Geometry: final body of the model. Coordinates: model frame, mm. Face numbers are marked on the shaded views. A direction names the side the tool comes from. Give positions to 0.01 mm unless a question says otherwise; leave off trailing zeros. Write each loop counter-clockwise with the first axis right and the second up, starting at its lowest first coordinate (ties: lowest second). Pieces come first, ordered by that corner, then holes. Notation, with made-up numbers: M -19,-21.75 L 29,-21.75 A22 ccw 29,-11.75 Z; hole C 46,48.5 d5. An arc over 180 degrees is marked long. Answer as a JSON object with one key per item and string values.
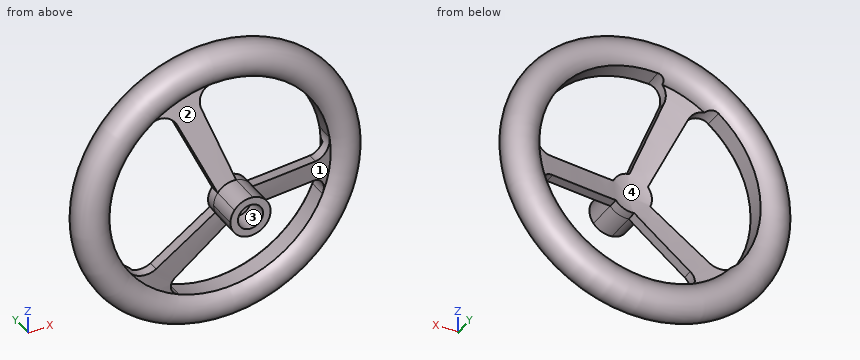
from build123d import *

# Parameters (mm, degrees)
CUT_EXTRUDE1_DEPTH = 218.993055499


with BuildPart() as part:
    # Sketch1 → Revolve1 (revolve)
    with BuildSketch(Plane.XY, mode=Mode.PRIVATE) as revolve1_sk:
        with BuildLine():
            Line((20, -100.740243091), (20, -69.715325618))
            Line((20, -69.715325618), (110.198752068, -44.459675039))
            ThreePointArc((110.198752068, -44.459675039), (141.851870345, -30.404499927), (107.502452813, -34.830034842))
            Line((107.502452813, -34.830034842), (0, -64.930721629))
            Line((0, -64.930721629), (0, -78.058110007))
            Line((0, -78.058110007), (12.5, -78.058110007))
            Line((12.5, -78.058110007), (12.5, -100.740243091))
            Line((12.5, -100.740243091), (20, -100.740243091))
        make_face()
    revolve(revolve1_sk.sketch.rotate(Axis((0, 122.203800038, 0), (0, -1, 0)), 180), axis=Axis((0, 122.203800038, 0), (0, -1, 0)))

    # Sketch3 → Cut-Extrude1 (cut, through all)
    with BuildSketch(Plane.XZ.offset(100.740243091)):
        with BuildLine():
            Line((-15.982116295, 12.023807996), (-45.159681095, 80.612688819))
            ThreePointArc((-45.159681095, 80.612688819), (-55.246837021, 89.273395117), (-68.253125072, 86.51748884))
            ThreePointArc((-68.253125072, 86.51748884), (-109.03897279, 15.945763394), (-90.169598509, -63.349889203))
            ThreePointArc((-90.169598509, -63.349889203), (-78.581603296, -69.711168161), (-66.461068877, -64.43479171))
            Line((-66.461068877, -64.43479171), (-18.403981322, -7.82901472))
            ThreePointArc((-18.403981322, -7.82901472), (-19.852822716, 2.421865027), (-15.982116295, 12.023807996))
        make_face()
        with BuildLine():
            Line((15.982116295, -12.023807996), (89.970611905, -21.04973607))
            ThreePointArc((89.970611905, -21.04973607), (101.087630383, -28.341543009), (102.04423972, -41.602140538))
            ThreePointArc((102.04423972, -41.602140538), (43.137382604, -101.40478874), (-40.799780672, -102.36768462))
            ThreePointArc((-40.799780672, -102.36768462), (-49.689609543, -92.481861898), (-47.232795837, -79.415775465))
            Line((-47.232795837, -79.415775465), (-2.421865027, -19.852822716))
            ThreePointArc((-2.421865027, -19.852822716), (7.82901472, -18.403981322), (15.982116295, -12.023807996))
        make_face()
        with BuildLine():
            Line((2.421865027, 19.852822716), (-21.185241198, 90.169588344))
            ThreePointArc((-21.185241198, 90.169588344), (-19.455713432, 103.249492349), (-8.062704922, 109.903401888))
            ThreePointArc((-8.062704922, 109.903401888), (69.001859108, 85.921524643), (109.052905743, 15.85019578))
            ThreePointArc((109.052905743, 15.85019578), (104.936446564, 3.208466781), (92.392476932, -1.196913354))
            Line((92.392476932, -1.196913354), (18.403981322, 7.82901472))
            ThreePointArc((18.403981322, 7.82901472), (12.023807996, 15.982116295), (2.421865027, 19.852822716))
        make_face()
    extrude(amount=-CUT_EXTRUDE1_DEPTH, mode=Mode.SUBTRACT)


solid = part.part
1) Contact query for flat-ended pins moving along their axis: P1, Ø3, axis at x = -10.5, y = -79.5, coming from the +Z side; P2, Ø5, axis at x = -88, y = -26, coming from the +Z side; P3, Ø3, axis at y = -46.5, z = 89, coming from the +X side. Output: stop coordinate, or through.
Geometry check:
{"P1": "stops at z = 17.86", "P2": "stops at z = 111.42", "P3": "stops at x = 107.83"}
2) Cut plane B-B on z = -60. Give the number of separate pieces and of enclosed holes in the cut face, and give its area (3 significant figures).
Geometry check:
{"separate pieces": "3", "enclosed holes": "0", "area": "2,430 mm2"}
3) Set-up query: the marked faces 3 and 4. Return all of +Z, -Z, +X, -X, +Y, -Y with unobstructed straight access to the full face (end or side cutting, diameter ignored); none if empty.
Geometry check:
{"face 3": "-Y", "face 4": "+Y"}
4) Pull-direction query (X, two-part tool) for the marked faces 1 and 2; classes: pulls with the +X half, pulls with the -X half, needs draft (parallel to the pull), parting line crosses it, or undercut.
Geometry check:
{"face 1": "undercut", "face 2": "undercut"}
5) Line query: line 1 (Z direction, x = 0, y = -86.25); line 2 (X direction, y = -24, z = 51); line 3 (Y direction, x = -66.5, z = 105.5). Output: solid intervals per line, ascending. Write a range as from..to.
Geometry check:
{"line 1": "z = -20..-12.5, 12.5..20", "line 2": "x = -128.78..-99.14, 99.14..128.78", "line 3": "y = -52.62..-17.63"}
6) Cut plane A-A on y = -93.5. Return loops of the section in (x, z), and give its area (3 significant figures).
Geometry check:
{"outline": "C 0,0 d40; hole C 0,0 d25", "area": "766 mm2"}
